Autodesk Inventor part; units mm, degrees
ref_plane "YZ Plane" through (0, 0, 0) normal (1, 0, 0) x (0, 1, 0)
ref_plane "XZ Plane" through (0, 0, 0) normal (0, 1, 0) x (-1, 0, 0)
ref_plane "XY Plane" through (0, 0, 0) normal (0, 0, 1) x (1, 0, 0)
sketch "Sketch1" plane through (0, 0, 0) normal (1, 0, 0) x (0, 1, 0)
  line L0 (0, 0) -> (10.16, 0)
  line L1 (10.16, 0) -> (10.16, -7.62)
  line L2 (0, -7.62) -> (0, 0)
  arc A0 (10.16, -7.62) -> (0, -7.62) centre (5.08, -12.7876) ccw
  line L3 (10.16, 0) -> (6.0753, 0)
  line L4 (5.08, 0) -> (5.08, -12.7876) construction
  dimension "d1" = 10.16
  dimension "d2" = 7.62
revolve "Revolution1" add sketch "Sketch1" angle 360 about axis through (0, 10.16, 0) along (0, -1, 0)
sketch "Sketch2" plane through (0, 0, 0) normal (0, -1, 0) x (1, 0, 0)
  circle A0 centre (0, 0) radius 5.5
  dimension "d3" = 11
extrude "Extrusion1" cut sketch "Sketch2" against normal blind 1.4
sketch "Sketch3" plane through (0, 1.4, 0) normal (0, -1, 0) x (1, 0, 0)
  circle A0 centre (0, 0) radius 3.925
  dimension "d6" = 7.85
extrude "Extrusion2" cut sketch "Sketch3" against normal through all
properties part number "top pulley"
Work out the finished part from the listing and answer in its coordinate system (mm). A direction names the side the tool comes from. Coordinates: 2 decimals unless noted, no trailing zeros. Write each loop counter-clockwise with the first axis right and the second up, starting at its lowest first coordinate (ties: lowest second). Pieces come first, ordered by that corner, then holes.
1. For faces 1 (the cylindrical face through (-2.893, 5.719, 2.653)), 2 (the cylindrical face through (-1.19, 0.69, -5.37)), determine the directions among +Z, -Z, +X, -X, +Y, -Y from which every point of the face is accessible in a straight line to the end or side of a thin tool.
Results list:
face 1: +Y, -Y
face 2: -Y
2. The part is cut by section A-A, the plane x = 0. Write down the section's boundary in (y, z) (3 decimals).
Results list:
outline: (0, -7.62) arc R7.246 cw to (10.16, -7.62) - (10.16, -3.925) - (1.4, -3.925) - (1.4, -5.5) - (0, -5.5) - close; (0, 5.5) - (1.4, 5.5) - (1.4, 3.925) - (10.16, 3.925) - (10.16, 7.62) arc R7.246 cw to (0, 7.62) - close
3. The part is cut by section D-D, the plane y = 6.5. Write down the section's boundary in (x, z) (3 decimals), and give its area (3 significant figures).
Results list:
outline: circle Ø11.363 at (0, 0); hole circle Ø7.85 at (0, 0)
area: 53.0 mm2
4. For a pull along Z with two mould halves and no side action, classify faces 3 (the flat face through (4, 0, -4)), 4 (the flat face through (-1, 1.4, 4)) as +Z half, -Z half, draft (parallel to the pull), parting line (faces both ways), or undercut.
Results list:
face 3: draft
face 4: undercut
5. Flat-ended cylindrical pins translate along their axes: pin 1 (1 mm diameter, centred on y = 8, z = -0.5, fed in from -X); pin 2 (6 mm diameter, centred on y = 2.5, z = 2, fed in from +X); pin 3 (6.5 mm diameter, centred on x = 0, z = 0, fed in from -Y); pin 4 (3 mm diameter, centred on y = 7, z = 2, fed in from +X). Find the tip coordinate at first contact, or state that the pin passes through.
Results list:
pin 1: stops at x = -6.38
pin 2: stops at x = 7.61
pin 3: passes through
pin 4: stops at x = 6.18
6. Consider line 1 along Z through (x, y) = (-0.25, 6.25); line 2 along Y through (x, z) = (4, 1.75); line 3 along Z through (x, y) = (0, 7) (3 decimals). Determine where each line is inside the solid, lowest interval first.
Results list:
line 1: z = -5.63 to -3.92, 3.92 to 5.63
line 2: y = 1.4 to 10.16
line 3: z = -5.8 to -3.925, 3.925 to 5.8
7. The part is cut by section C-C, the plane y = 5.25. Write down the section's boundary in (x, z) (3 decimals).
Results list:
outline: circle Ø11.086 at (0, 0); hole circle Ø7.85 at (0, 0)
8. The part is cut by section B-B, the plane z = 0. Write down the section's boundary in (x, y) (3 decimals).
Results list:
outline: (-7.62, 0) - (-5.5, 0) - (-5.5, 1.4) - (-3.925, 1.4) - (-3.925, 10.16) - (-7.62, 10.16) arc R7.246 cw to start; (3.925, 1.4) - (5.5, 1.4) - (5.5, 0) - (7.62, 0) arc R7.246 cw to (7.62, 10.16) - (3.925, 10.16) - close
